Source: CAD feature listing. Evaluate the final solid. Frame: model axes, mm. A direction names the side the tool comes from. Give positions to 0.01 mm unless a question says otherwise; leave off trailing zeros. Loops run counter-clockwise (first coordinate to the right, second up) from the corner with the lowest first, then second, coordinate; pieces in that order, holes last. Notation, with made-up numbers: M -13,72.25 L 40,72.25 A30 cw 40,101.25 Z; hole C 38.25,78 d1. An arc over 180 degrees is marked long. Answer in a Markdown table with one row per item.
```python
from build123d import *

# Parameters (mm, degrees)
BOSS_EXTRUDE1_DEPTH      = 9
BOSS_EXTRUDE1_DEPTH_BACK = 9
SKETCH1_R                = 16.05
BOSS_EXTRUDE2_DEPTH      = 2
BOSS_EXTRUDE2_DEPTH_BACK = 2
SKETCH2_R                = 11.05
SKETCH3_R                = 1.4
CUT_EXTRUDE1_DEPTH       = 58.158573285
FILLET1_R                = 2
FILLET2_R                = 1


with BuildPart() as part:
    # Sketch1 → Boss-Extrude1 (new, two sides: drawn at the far end of the back side and taken through both)
    with BuildSketch(Plane.XY.offset(-BOSS_EXTRUDE1_DEPTH_BACK)):
        with BuildLine():
            Line((0, 21.05), (-50, 21.05))
            Line((-50, 21.05), (-50, -21.05))
            Line((-50, -21.05), (0, -21.05))
            ThreePointArc((0, -21.05), (21.05, 0), (0, 21.05))
        make_face()
        Circle(SKETCH1_R, mode=Mode.SUBTRACT)
    extrude(amount=BOSS_EXTRUDE1_DEPTH + BOSS_EXTRUDE1_DEPTH_BACK)

    # Sketch2 → Boss-Extrude2 (add, two sides: drawn at the far end of the back side and taken through both)
    with BuildSketch(Plane(origin=(0, 0, 0), x_dir=(-1, 0, 0), z_dir=(0, 0, -1)).offset(-BOSS_EXTRUDE2_DEPTH_BACK)):
        with BuildLine():
            Line((0, -21.05), (50, -21.05))
            Line((50, -21.05), (50, 21.05))
            Line((50, 21.05), (0, 21.05))
            ThreePointArc((0, 21.05), (-21.05, 0), (0, -21.05))
        make_face()
        with Locations(Location((0, 0, 0), (0, 0, 180))):
            Circle(SKETCH2_R, mode=Mode.SUBTRACT)
    extrude(amount=BOSS_EXTRUDE2_DEPTH + BOSS_EXTRUDE2_DEPTH_BACK)

    # Sketch3 → Cut-Extrude1 (cut, through all)
    with BuildSketch(Plane.XY.offset(9)):
        with Locations((-45, 16.05)):
            Circle(SKETCH3_R)
        with Locations((-20, 16.05)):
            Circle(SKETCH3_R)
        with Locations((-20, -16.05)):
            Circle(SKETCH3_R)
        with Locations((-45, -16.05)):
            Circle(SKETCH3_R)
    extrude(amount=-CUT_EXTRUDE1_DEPTH, mode=Mode.SUBTRACT)

    # Fillet1
    fillet1_edges = [part.edges().sort_by_distance(p)[0] for p in [
        (-50, -21.05, 0),
        (-50, 21.05, 0),
    ]]
    fillet(fillet1_edges, radius=FILLET1_R)

    # Fillet2
    fillet2_edges = [part.edges().sort_by_distance(p)[0] for p in [
        (-16.05, 0, -9),
        (-16.05, 0, 9),
    ]]
    fillet(fillet2_edges, radius=FILLET2_R)


solid = part.part
```
1) Section A-A, the plane x = -20. Return loops of the section in (y, z).
Reply:
| item | result |
|---|---|
| outline | M -21.05,-9 L -17.45,-9 L -17.45,9 L -21.05,9 Z; M -14.65,-9 L 14.65,-9 L 14.65,9 L -14.65,9 Z; M 17.45,-9 L 21.05,-9 L 21.05,9 L 17.45,9 Z |
2) Section C-C, the plane z = 0. Return loops of the section in (x, y).
Reply:
| item | result |
|---|---|
| outline | M -50,-19.05 A2 ccw -48,-21.05 L 0,-21.05 A21.05 ccw 0,21.05 L -48,21.05 A2 ccw -50,19.05 Z; hole C -45,-16.05 d2.8; hole C -45,16.05 d2.8; hole C -20,-16.05 d2.8; hole C -20,16.05 d2.8; hole C 0,0 d22.1 |
3) Pin query (flat end, axial travel): pin 1 Ø1.7 at (x, y) = (-45, 16.05) entering from +Z; pin 2 Ø3.5 at (x, y) = (-45, -16.05) entering from -Z; pin 3 Ø8 at (x, y) = (-4.5, -9.5) entering from -Z; pin 4 Ø5 at (x, z) = (12.5, 3.5) entering from +Y. Return the tip coordinate at first contact, or that it passes through.
Reply:
| item | result |
|---|---|
| pin 1 | passes through |
| pin 2 | stops at z = -9 |
| pin 3 | stops at z = -2 |
| pin 4 | stops at y = 18.52 |
4) Material intervals for L1, parallel to Y at x = -45, z = 1.25; L2, parallel to X at y = -0.5, z = 2.5; L3, parallel to Y at x = -21, z = 4.25, sorted ascending.
Reply:
| item | result |
|---|---|
| L1 | y = -21.05 to -17.45, -14.65 to 14.65, 17.45 to 21.05 |
| L2 | x = -50 to -16.04, 16.04 to 21.04 |
| L3 | y = -21.05 to -17.03, -15.07 to 15.07, 17.03 to 21.05 |
5) Set-up query: faces 4 (the flat face through (-3, 11, -2)), 5 (the cylindrical face through (-20.303, 14.683, 0.126)), 6 (the flat face through (-3, 11, 2)). Return all of +Z, -Z, +X, -X, +Y, -Y with unobstructed straight access to the full face (end or side cutting, diameter ignored); none if empty.
Reply:
| item | result |
|---|---|
| face 4 | -Z |
| face 5 | +Z, -Z |
| face 6 | +Z |
6) Section B-B, the plane z = 3. Return loops of the section in (x, y).
Reply:
| item | result |
|---|---|
| outline | M -50,-19.05 A2 ccw -48,-21.05 L 0,-21.05 A21.05 ccw 0,21.05 L -48,21.05 A2 ccw -50,19.05 Z; hole C -45,-16.05 d2.8; hole C -45,16.05 d2.8; hole C -20,-16.05 d2.8; hole C -20,16.05 d2.8; hole C 0,0 d32.1 |
7) Pull-direction query (Y, two-part tool) for faces 1 (the cylindrical face through (-49.4, 20.48, 0.13)), 2 (the flat face through (-23, 0, -9)), 3 (the cylindrical face through (-12.737, -9.766, -5.042)); classes: released by +Y, released by -Y, zero draft, split by the parting line, or undercut.
Reply:
| item | result |
|---|---|
| face 1 | released by +Y |
| face 2 | zero draft |
| face 3 | undercut |
